Part print with two shaded views. Sizes in mm from the minimum x, y, z corner. Round coordinates to 2 decimals unless told otherwise and drop trailing zeros. Loops run counter-clockwise (first coordinate to the right, second up) from the corner with the lowest first, then second, coordinate; pieces in that order, holes last. Notation, with made-up numbers: (59.25, 66.25) -> (91.25, 66.25) arc R29 cw to (91.25, 86.25) -> close; hole circle Ø1 at (61.25, -15). An arc over 180 degrees is marked (long way). Answer as a JSON object with one key per item and string values. Group by question number.
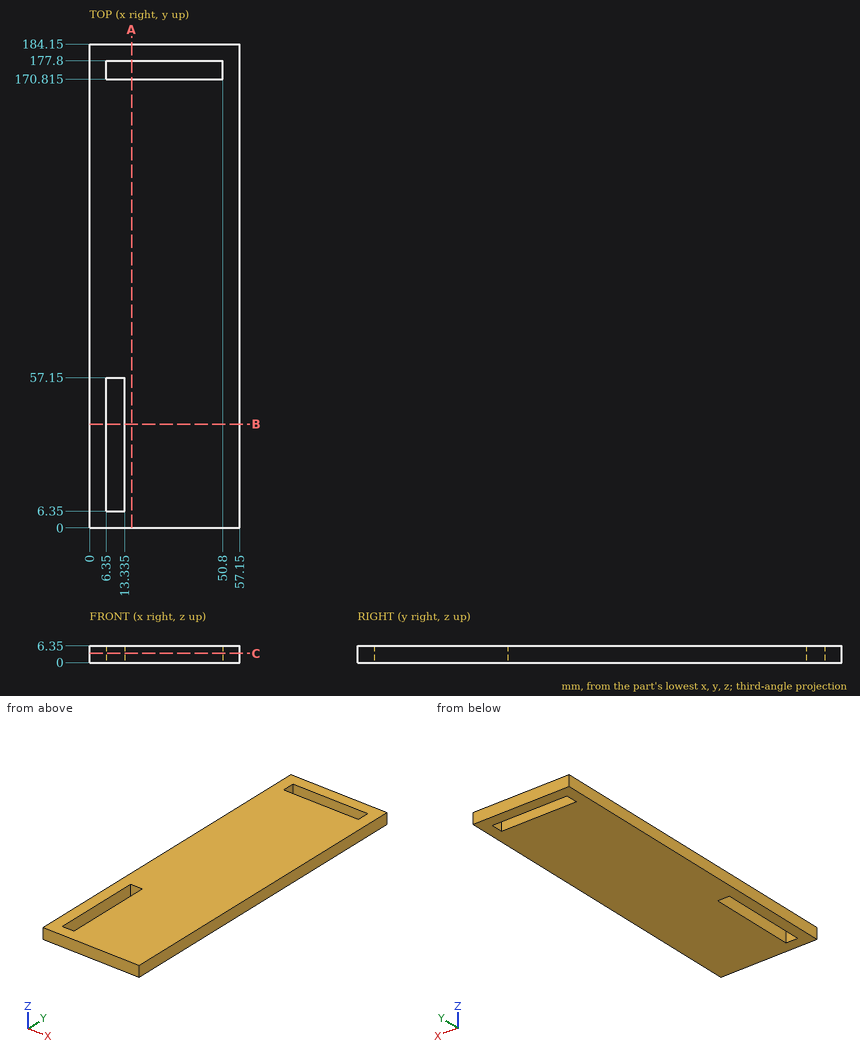
Item 1: Band-saw the part on C-C, the plane z = 3.5. List the corners of the cut face in (x, y) (3 decimals), plus the area to 3 significant figures.
Item 2: Drill centre lines: line 1 (Y direction, x = 10.5, z = 2) (3 decimals); line 2 (Y direction, x = 21, z = 0.75) (3 decimals); line 3 (X direction, y = 42.5, z = 5) (3 decimals). Where is each one in solid material? Low to high.
Item 3: Band-saw the part on B-B, the plane y = 39.5. List the corners of the cut face in (x, z) (3 decimals), plus the area to 3 significant figures.
Item 4: Drop a flat-ended pin along its axis: pin 1 Ø3 at (y, z) = (27, 4) entering from -X. Give the stop position or say it passes through.
Item 5: Band-saw the part on A-A, the plane x = 16. List the corners of the cut face in (y, z) (3 decimals).
Entries:
{
 "1": {"outline": "(0, 0) -> (57.15, 0) -> (57.15, 184.15) -> (0, 184.15) -> close; hole (6.35, 6.35) -> (13.335, 6.35) -> (13.335, 57.15) -> (6.35, 57.15) -> close; hole (6.35, 170.815) -> (50.8, 170.815) -> (50.8, 177.8) -> (6.35, 177.8) -> close", "area": "9,860 mm²"},
 "2": {"line 1": "0 to 6.35, 57.15 to 170.815, 177.8 to 184.15", "line 2": "0 to 170.815, 177.8 to 184.15", "line 3": "0 to 6.35, 13.335 to 57.15"},
 "3": {"outline": "(0, 0) -> (6.35, 0) -> (6.35, 6.35) -> (0, 6.35) -> close; (13.335, 0) -> (57.15, 0) -> (57.15, 6.35) -> (13.335, 6.35) -> close", "area": "319 mm²"},
 "4": {"pin 1": "x = 0"},
 "5": {"outline": "(0, 0) -> (170.815, 0) -> (170.815, 6.35) -> (0, 6.35) -> close; (177.8, 0) -> (184.15, 0) -> (184.15, 6.35) -> (177.8, 6.35) -> close"}
}
